Could you check a few things on this drawing? It's one solid part, dimensions in mm from its lowest x, y, z. Give positions to 0.01 mm unless a question says otherwise; leave off trailing zeros. Order: outer loops, then holes, each group sorted by start corner. A loop starts at its lowest first (then second) coordinate and runs counter-clockwise, first axis right, second up. Notation, with made-up numbers: M 27,-3 L 50,-3 A7 cw 50,6 Z; hole C 1.25,-39.5 d1. An arc over 180 degrees is marked long. One line per item, written item: value. Start each with the question number.
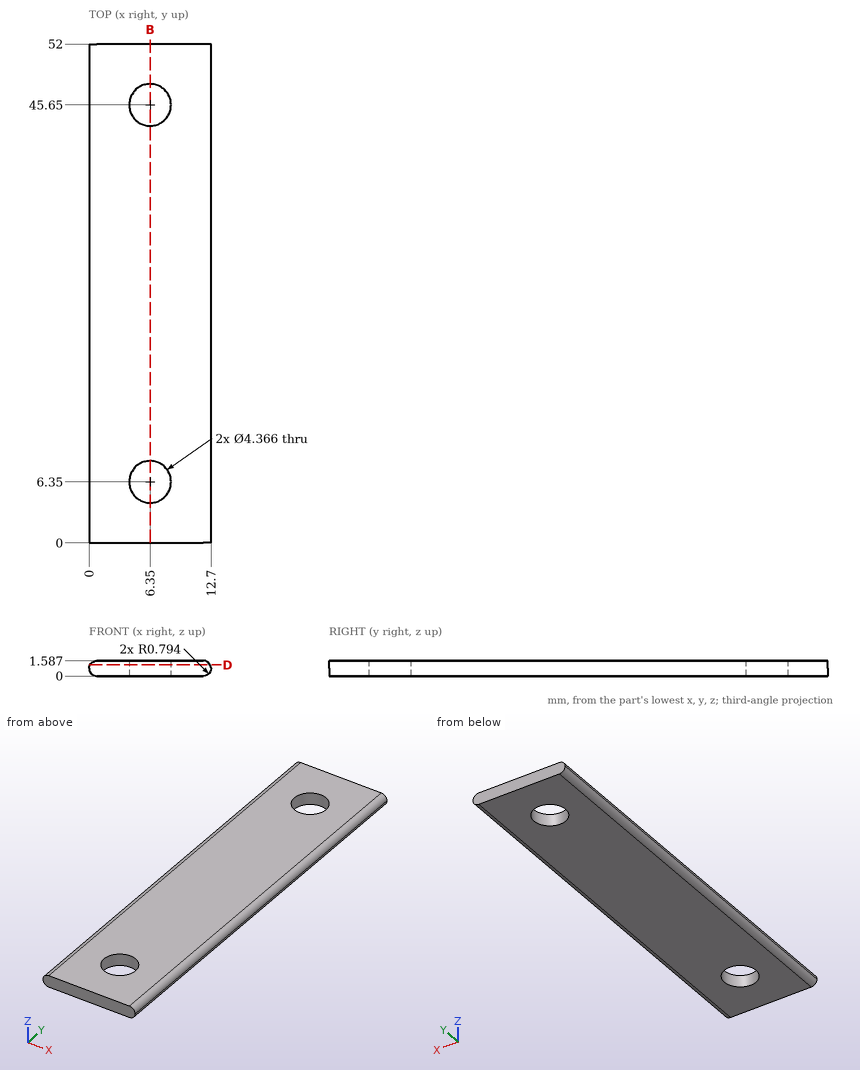
Item 1: Will this pin go through, and if not, where does the flat tip stop? P1, Ø5.5, axis at x = 6.35, y = 6.35, coming from the -Z side.
Item 2: Please list where these lines run through material, in increasing order: probe 1 along Y at (x, z) = (6.35, 0.45); probe 2 along Y at (x, z) = (4.75, 1.35) (1 decimal); probe 3 along X at (y, z) = (41, 0.75). Write a range as [from, to].
Item 3: I want a section at D-D on z = 1.15. Count the separate pieces of the cut face and the enclosed holes in it, plus the area to 3 significant figures.
Item 4: I want a section at B-B on x = 6.35. Write out the boundary of the cut face in (y, z).
Answer below:
1. P1: stops at z = 0
2. probe 1: y = [0, 4.17], [8.53, 43.47], [47.83, 52]
2. probe 2: y = [0, 4.9], [7.8, 44.2], [47.1, 52]
2. probe 3: x = [0, 12.7]
3. separate pieces: 1
3. enclosed holes: 2
3. area: 622 mm²
4. outline: M 0,0 L 4.17,0 L 4.17,1.59 L 0,1.59 Z; M 8.53,0 L 43.47,0 L 43.47,1.59 L 8.53,1.59 Z; M 47.83,0 L 52,0 L 52,1.59 L 47.83,1.59 Z
